```python
from build123d import *

# Parameters (mm, degrees)
SKETCH_1_R      = 60
SKETCH_1_R_2    = 26
EXTRUDE_1_DEPTH = 20
FILLET_1_R      = 1
SKETCH_2_R      = 26
SKETCH_2_R_2    = 23
EXTRUDE_2_DEPTH = 3


with BuildPart() as part:
    # 草图1 → 凸台-拉伸1 (new body)
    with BuildSketch(Plane(origin=(0, 0, 0), x_dir=(1, 0, 0), z_dir=(0, 1, 0))):
        Circle(SKETCH_1_R)
        Circle(SKETCH_1_R_2, mode=Mode.SUBTRACT)
    extrude(amount=EXTRUDE_1_DEPTH)

    # 圆角1
    fillet_1_edges = [part.edges().sort_by_distance(p)[0] for p in [
        (-60, 0, 0),
        (-60, 20, 0),
    ]]
    fillet(fillet_1_edges, radius=FILLET_1_R)

    # 草图2 → 凸台-拉伸2 (add)
    with BuildSketch(Plane.XZ):
        Circle(SKETCH_2_R)
        Circle(SKETCH_2_R_2, mode=Mode.SUBTRACT)
    extrude(amount=-EXTRUDE_2_DEPTH)


solid = part.part
```
Input: part model. Units: mm. Frame: model coordinates. A direction names the side the tool comes from. Give positions to 0.01 mm unless a question says otherwise; leave off trailing zeros. Order: outer loops, then holes, each group sorted by start corner. A loop starts at its lowest first (then second) coordinate and runs counter-clockwise, first axis right, second up.
1. Reachability of faces 4 (the cylindrical face through (-20.633, 11.381, 15.821)), 5 (the flat face through (25, 20, 12)) from +Z, -Z, +X, -X, +Y, -Y: full face, straight path, thin tool, end or side. Return the list, or none.
Derived:
face 4: +Y
face 5: +Z, -Z, +X, -X, +Y
2. Section C-C on y = 6.75. Return the cut outline in (x, z), and give its area (3 significant figures).
Derived:
outline: circle Ø120 at (0, 0); hole circle Ø52 at (0, 0)
area: 9,190 mm2
3. Pin query (flat end, axial travel): pin 1 (6 mm diameter, centred on x = -19.5, y = 17.5, fed in from +Z); pin 2 (8 mm diameter, centred on x = -22.5, y = 6.5, fed in from -Z); pin 3 (10 mm diameter, centred on x = 20.5, y = 16.5, fed in from +Z). Return the tip coordinate at first contact, or that it passes through.
Derived:
pin 1: stops at z = 57.69
pin 2: stops at z = -57.08
pin 3: stops at z = 57.96
4. Section A-A on z = 0. Return the cut outline in (x, y).
Derived:
outline: (-60, 1) arc R1 ccw to (-59, 0) - (-23, 0) - (-23, 3) - (-26, 3) - (-26, 20) - (-59, 20) arc R1 ccw to (-60, 19) - close; (23, 0) - (59, 0) arc R1 ccw to (60, 1) - (60, 19) arc R1 ccw to (59, 20) - (26, 20) - (26, 3) - (23, 3) - close
5. Material intervals for L1, parallel to X at y = 7, z = 0; L2, parallel to Z at x = 0, y = 0.85, sorted ascending.
Derived:
L1: x = -60 to -26, 26 to 60
L2: z = -59.99 to -23, 23 to 59.99
6. Mould query, pull axis Z, two halves, no side actions, for faces 1 (the flat face through (-1, 0, -25)), 2 (the cylindrical face through (-59.94, 9.87, -2.64)), 3 (the flat face through (10, 3, -21)). Classes: released by +Z, released by -Z, zero draft, split by the parting line, or undercut.
Derived:
face 1: zero draft
face 2: split by the parting line
face 3: undercut
7. Section B-B on x = 0. Return the cut outline in (y, z).
Derived:
outline: (0, -59) arc R1 ccw to (1, -60) - (19, -60) arc R1 ccw to (20, -59) - (20, -26) - (3, -26) - (3, -23) - (0, -23) - close; (0, 23) - (3, 23) - (3, 26) - (20, 26) - (20, 59) arc R1 ccw to (19, 60) - (1, 60) arc R1 ccw to (0, 59) - close
